The drawing under review shows one solid part. Ordinate dimensions are in mm from its lowest x, y, z. A direction names the side the tool comes from. Round coordinates to 2 decimals unless told otherwise and drop trailing zeros. Write each loop counter-clockwise with the first axis right and the second up, starting at its lowest first coordinate (ties: lowest second). Pieces come first, ordered by that corner, then holes. Notation, with made-up numbers: (82.25, -35.5) -> (86.25, -35.5) arc R23 cw to (86.25, -16.5) -> close; hole circle Ø3 at (35, 25.25). An arc over 180 degrees is marked (long way). Write item = value, one per line. Start each with the question number.
Item 1: Add section C-C, the plane x = 3.75. State the section outline as (y, z) points.
Item 2: Mouldability with a two-part tool opening along X and no side actions: class the marked faces 1, 2, 3 and 4 as released by +X, released by -X, zero draft, split by the parting line, or undercut.
Item 3: To check wall thickness, follow L1, parallel to X at y = 7.75, z = 5.5; L2, parallel to X at y = 4.25, z = 0.75; L3, parallel to Y at x = 8.5, z = 5.5. State the ranges of each line that lie inside material, in increasing order.
Item 4: Add section A-A, the plane z = 4. State the section outline as (x, y) points.
Item 5: For pin 1 Ø1.5 at (x, y) = (12, 11.5) entering from -Z, flat-tipped, find the tip position at first contact; note if it passes through.
Item 6: Add section D-D, the plane y = 3. State the section outline as (x, z) points (1 decimal).
Item 7: Add section B-B, the plane y = 14.5. State the section outline as (x, z) points.
Item 8: Machinability: for the marked faces 5, 6 and 7, which of the approach directions +Z, -Z, +X, -X, +Y, -Y give a long, thin tool a straight path to every point of the face, cutting with its end or side? Answer none if there is none.
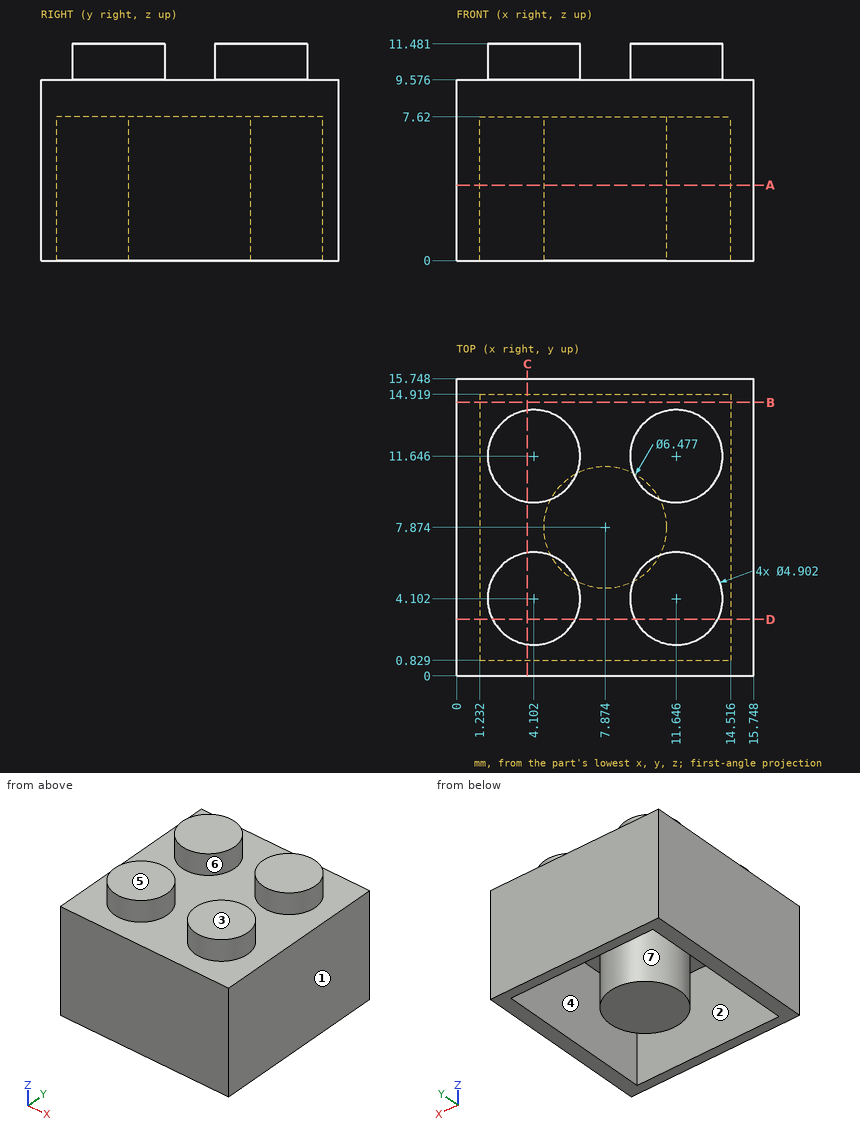
Result set:
q1.outline = (0, 0) -> (0.83, 0) -> (0.83, 7.62) -> (14.92, 7.62) -> (14.92, 0) -> (15.75, 0) -> (15.75, 9.58) -> (14.07, 9.58) -> (14.07, 11.48) -> (9.22, 11.48) -> (9.22, 9.58) -> (6.53, 9.58) -> (6.53, 11.48) -> (1.68, 11.48) -> (1.68, 9.58) -> (0, 9.58) -> close
q2.face_1 = released by +X
q2.face_2 = undercut
q2.face_3 = zero draft
q2.face_4 = undercut
q3.L1 = 0 to 1.23, 4.64 to 11.11, 14.52 to 15.75
q3.L2 = 0 to 1.23, 14.52 to 15.75
q3.L3 = 0 to 0.83, 4.7 to 11.05, 14.92 to 15.75
q4.outline = (0, 0) -> (15.75, 0) -> (15.75, 15.75) -> (0, 15.75) -> close; circle Ø6.48 at (7.87, 7.87); hole (1.23, 0.83) -> (14.52, 0.83) -> (14.52, 14.92) -> (1.23, 14.92) -> close
q5.pin_1 = 7.62
q6.outline = (0, 0) -> (1.2, 0) -> (1.2, 7.6) -> (14.5, 7.6) -> (14.5, 0) -> (15.7, 0) -> (15.7, 9.6) -> (13.8, 9.6) -> (13.8, 11.5) -> (9.5, 11.5) -> (9.5, 9.6) -> (6.3, 9.6) -> (6.3, 11.5) -> (1.9, 11.5) -> (1.9, 9.6) -> (0, 9.6) -> close
q7.outline = (0, 0) -> (1.23, 0) -> (1.23, 7.62) -> (14.52, 7.62) -> (14.52, 0) -> (15.75, 0) -> (15.75, 9.58) -> (0, 9.58) -> close
q8.face_5 = +Z, +X, -X, +Y, -Y
q8.face_6 = +Z
q8.face_7 = -Z
